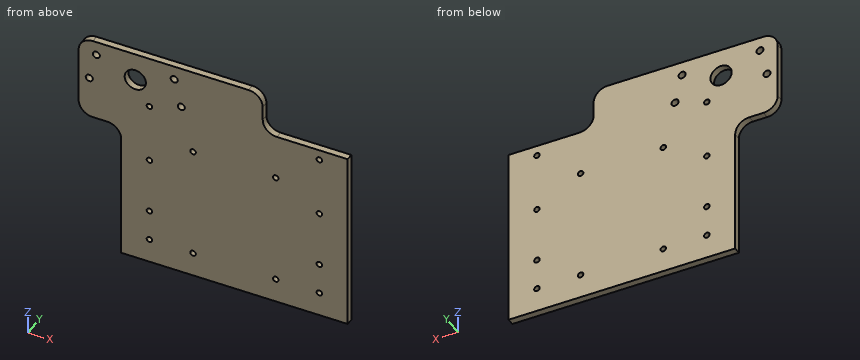
Autodesk Inventor part; units mm, degrees
ref_plane "YZ Plane" through (0, 0, 0) normal (1, 0, 0) x (0, 1, 0)
ref_plane "XZ Plane" through (0, 0, 0) normal (0, 1, 0) x (-1, 0, 0)
ref_plane "XY Plane" through (0, 0, 0) normal (0, 0, 1) x (1, 0, 0)
sketch "Sketch1" plane through (0, 0, 0) normal (0, 1, 0) x (-1, 0, 0)
  line L0 (0, 0) -> (203.2, 0)
  line L1 (203.2, 0) -> (203.2, 114.3)
  line L2 (76.2, 165.1) -> (0, 165.1)
  line L3 (0, 165.1) -> (0, 0)
  line L4 (76.2, 165.1) -> (76.2, 190.5)
  line L5 (88.9, 203.2) -> (228.6, 203.2)
  arc A0 (63.5, 165.1) -> (76.2, 177.8) centre (63.5, 177.8) ccw
  arc A1 (241.3, 190.5) -> (228.6, 203.2) centre (228.6, 190.5) ccw
  arc A2 (88.9, 203.2) -> (76.2, 190.5) centre (88.9, 190.5) ccw
  line L6 (146.05, 0) -> (57.15, 0)
  line L7 (215.9, 127) -> (228.6, 127)
  line L8 (241.3, 139.7) -> (241.3, 190.5)
  arc A3 (215.9, 127) -> (203.2, 114.3) centre (215.9, 114.3) ccw
  arc A4 (228.6, 127) -> (241.3, 139.7) centre (228.6, 139.7) ccw
  point P0 (76.2, 203.2)
  point P1 (241.3, 127)
  dimension "d64" = 38.1
  dimension "d67" = 12.7
  dimension "d69" = 12.7
  dimension "d105" = 76.2
  dimension "d106" = 12.7
  dimension "d108" = 203.2
  dimension "d109" = 127
  dimension "d110" = 165.1
  dimension "d111" = 38.1
extrude "Plate2" add sketch "Sketch1" along normal blind 6.35
sketch "Sketch5" plane through (0, 6.35, 0) normal (0, 1, 0) x (1, 0, 0)
  line L0 (-203.2, -114.3) -> (-203.2, 0)
  line L1 (0, 0) -> (0, -165.1)
  line L2 (-203.2, 0) -> (0, 0)
  point P0 (-203.2, -165.1)
  point P1 (-177.8, -22.225)
  point P2 (-25.4, -22.225)
  point P3 (-25.4, -155.575)
  point P4 (-177.8, -155.575)
  point P5 (-177.8, -50.8)
  point P6 (-177.8, -101.6)
  point P7 (-25.4, -50.8)
  point P8 (-25.4, -101.6)
  point P9 (-203.2, -203.2)
  point P10 (-138.684, -22.225)
  point P11 (-64.516, -22.225)
  point P12 (-138.684, -123.825)
  point P13 (-64.516, -123.825)
  dimension "d27" = 25.4
  dimension "d28" = 25.4
  dimension "d30" = 133.35
  dimension "d62" = 22.225
  dimension "d89" = 50.8
  dimension "d90" = 50.8
  dimension "d91" = 25.4
  dimension "d93" = 152.4
  dimension "d94" = 25.4
  dimension "d147" = 64.516
  dimension "d148" = 64.516
  dimension "d149" = 101.6
hole "Hole2" at (-177.8, 6.35, 22.225) at (-25.4, 6.35, 22.225) at (-25.4, 6.35, 155.575) at (-177.8, 6.35, 155.575) at (-177.8, 6.35, 101.6) at (-177.8, 6.35, 50.8) at (-25.4, 6.35, 50.8) at (-25.4, 6.35, 101.6) at (-64.516, 6.35, 123.825) at (-138.684, 6.35, 123.825) at (-138.684, 6.35, 22.225) at (-64.516, 6.35, 22.225) direction (0, -1, 0) diameter 4.9784 end through all
sketch "Sketch12" plane through (0, 6.35, 0) normal (0, 1, 0) x (1, 0, 0)
  line L0 (-241.3, -190.5) -> (-241.3, -139.7)
  line L1 (-228.6, -127) -> (-215.9, -127)
  point P0 (-203.2, -203.2)
  point P1 (-190.5, -177.8)
  dimension "d107" = 50.8
  dimension "d129" = 50.8
hole "Hole3" at (-190.5, 6.35, 177.8) direction (0, -1, 0) diameter 19.05 end through all
sketch "Sketch14" plane through (0, 6.35, 0) normal (0, 1, 0) x (1, 0, 0)
  circle A0 centre (-190.5, -177.8) radius 9.525
  point P0 (0, 0)
  point P1 (-225.425, -190.5)
  point P2 (-155.575, -190.5)
  point P3 (-149.225, -165.1)
  point P4 (-231.775, -165.1)
  dimension "d130" = 6.35
  dimension "d135" = 6.35
  dimension "d136" = 25.4
  dimension "d137" = 12.7
  dimension "d138" = 82.55
  dimension "d139" = 41.275
hole "Hole5" at (-225.425, 6.35, 190.5) at (-155.575, 6.35, 190.5) at (-149.225, 6.35, 165.1) at (-231.775, 6.35, 165.1) direction (0, -1, 0) diameter 6.35 end through all
equation "\"d102\" = Thickness"
equation "\"d145\" = Thickness"
equation "\"d106\" = d69"
equation "\"BendRadius\" = Thickness"
equation "\"BendReliefWidth\" = Thickness"
equation "\"BendReliefDepth\" = 0.5 * Thickness"
equation "\"CornerReliefSize\" = 4 * Thickness"
equation "\"MinimumRemnant\" = 2 * Thickness"
equation "\"TransitionRadius\" = BendRadius"
equation "\"JacobiRadiusSize\" = Thickness"
equation "\"GapSize\" = Thickness"
equation "\"d15\" = BendRadius"
equation "\"d16\" = BendRadius"
properties part number "backplate"
For this review, take the finished solid that the model builds, in its own axes (mm). Give positions to 0.01 mm unless a question says otherwise; leave off trailing zeros. Write each loop counter-clockwise with the first axis right and the second up, starting at its lowest first coordinate (ties: lowest second). Pieces come first, ordered by that corner, then holes. Notation, with made-up numbers: M 3,25 L 20,25 A21 cw 20,60 Z; hole C 46.25,-16.75 d11. An arc over 180 degrees is marked long. Answer as CSV lines item,"result".
1. Consider section C-C, the plane z = 61. Write out the cut boundary in (x, y).
Findings:
outline,"M -203.2,0 L 0,0 L 0,6.35 L -203.2,6.35 Z"
2. Consider section A-A, the plane x = -190.5. Write out the cut boundary in (y, z) (3 decimals), then the cut area to 3 significant figures.
Findings:
outline,"M 0,0 L 6.35,0 L 6.35,168.275 L 0,168.275 Z; M 0,187.325 L 6.35,187.325 L 6.35,203.2 L 0,203.2 Z"
area,"1,170 mm2"
3. For pin 1 (1 mm diameter, centred on y = 2.5, z = 60, fed in from -X); pin 2 (6.5 mm diameter, centred on x = -138.684, z = 123.825, fed in from -Y); pin 3 (1.9 mm diameter, centred on x = -27.5, y = 3.5, fed in from +Z); pin 4 (3 mm diameter, centred on x = -177.8, z = 50.8, fed in from -Y), all flat-tipped, find the tip position at first contact; note any pin that passes through.
Findings:
pin 1,"stops at x = -203.2"
pin 2,"stops at y = 0"
pin 3,"stops at z = 165.1"
pin 4,"passes through"
4. Wall thickness on line 1 (Z direction, x = -25.4, y = 4.5); line 2 (Z direction, x = -177.8, y = 3.25); line 3 (X direction, y = 4, z = 50.8): over which ranges is each line inside the solid? List them lowest first.
Findings:
line 1,"z = 0 to 19.74, 24.71 to 48.31, 53.29 to 99.11, 104.09 to 153.09, 158.06 to 165.1"
line 2,"z = 0 to 19.74, 24.71 to 48.31, 53.29 to 99.11, 104.09 to 153.09, 158.06 to 203.2"
line 3,"x = -203.2 to -180.29, -175.31 to -27.89, -22.91 to 0"
5. Consider section B-B, the plane y = 1.5. Count the separate pieces of the cut face and the enclosed holes in it, then the cut area to 3 significant figures.
Findings:
separate pieces,"1"
enclosed holes,"17"
area,"40,600 mm2"
